from build123d import *

# Parameters (mm, degrees)
SKETCH1_R           = 5
SKETCH1_R_2         = 2
SKETCH1_R_3         = 4
SKETCH1_R_4         = 11
BOSS_EXTRUDE1_DEPTH = 6


with BuildPart() as part:
    # Sketch1 → Boss-Extrude1 (new body)
    with BuildSketch(Plane.XY):
        with BuildLine():
            Line((-91.133667709, 81.856650449), (-59.395664216, 82.872754588))
            ThreePointArc((-59.395664216, 82.872754588), (-54.441095215, 84.371809376), (-50.89983999, 88.147313406))
            Line((-50.89983999, 88.147313406), (49.994476852, 276.580618392))
            Line((49.994476852, 276.580618392), (30.200235156, 308.463550017))
            ThreePointArc((30.200235156, 308.463550017), (26.424731127, 312.004805242), (21.384421113, 313.183870213))
            Line((21.384421113, 313.183870213), (-16.12412847, 311.983019868))
            Line((-16.12412847, 311.983019868), (-117.018445312, 123.549714881))
            ThreePointArc((-117.018445312, 123.549714881), (-118.197510284, 118.509404868), (-116.698455495, 113.554835867))
            Line((-116.698455495, 113.554835867), (-99.949481752, 86.576970646))
            ThreePointArc((-99.949481752, 86.576970646), (-96.173977723, 83.035715421), (-91.133667709, 81.856650449))
        make_face()
        with Locations((1.104829999, 270.012836125)):
            Circle(SKETCH1_R, mode=Mode.SUBTRACT)
        with Locations((-33.33250289, 254.422130449)):
            Circle(SKETCH1_R_2, mode=Mode.SUBTRACT)
        with Locations((11.628148729, 230.348497445)):
            Circle(SKETCH1_R_2, mode=Mode.SUBTRACT)
        with Locations((-28.022540924, 156.295659484)):
            Circle(SKETCH1_R_2, mode=Mode.SUBTRACT)
        with Locations((-43.879665152, 180.702169371)):
            Circle(SKETCH1_R_3, mode=Mode.SUBTRACT)
        with Locations((-72.983192543, 180.369292488)):
            Circle(SKETCH1_R_2, mode=Mode.SUBTRACT)
        with Locations((-76.464627777, 119.845498823)):
            Circle(SKETCH1_R_4, mode=Mode.SUBTRACT)
    extrude(amount=BOSS_EXTRUDE1_DEPTH)


solid = part.part
The model under review builds one solid part; all positions refer to its coordinate system, in mm. Coordinates: 2 decimals unless noted, no trailing zeros. Write each loop counter-clockwise with the first axis right and the second up, starting at its lowest first coordinate (ties: lowest second). Pieces come first, ordered by that corner, then holes. Notation, with made-up numbers: M 12.5,-12.5 L 54.5,-12.5 A19 cw 54.5,14.5 Z; hole C 2.25,47.25 d7. An arc over 180 degrees is marked long. Put each result on its own line as item: value.
1) Draft analysis for pull direction Z (two halves, no side actions). For faces 1 (the flat face through (-35, 199, 0)), 2 (the cylindrical face through (-65.973, 123.15, 2.958)), 3 (the flat face through (-35, 199, 6)), state which applies: released by +Z, released by -Z, zero draft, split by the parting line, or undercut.
Computed:
face 1: released by -Z
face 2: zero draft
face 3: released by +Z
2) Wall thickness on probe 1 along X at (y, z) = (231.5, 0.5); probe 2 along X at (y, z) = (116.5, 2.15); probe 3 along Y at (x, z) = (11, 1.4): over which ranges is each line inside the solid? List them lowest first. Write a range as [from, to].
Computed:
probe 1: x = [-59.22, 9.99], [13.26, 25.86]
probe 2: x = [-117.93, -86.94], [-65.99, -35.72]
probe 3: y = [203.75, 228.45], [232.25, 312.85]
3) Add section A-A on x = -43.5. Give the boundary of the cut face in (y, z) (3 decimals).
Computed:
outline: M 101.967,0 L 176.72,0 L 176.72,6 L 101.967,6 Z; M 184.684,0 L 260.855,0 L 260.855,6 L 184.684,6 Z
4) Clearance check with flat-ended pins moving along their axes: pin 1 Ø3 at (x, z) = (-54, 5) entering from -Y; pin 2 Ø1 at (x, z) = (6, 1.5) entering from -Y; pin 3 Ø1 at (y, z) = (106, 4) entering from -X. State where each tip first meets the part, or that it passes through.
Computed:
pin 1: stops at y = 83.8
pin 2: stops at y = 193.48
pin 3: stops at x = -112.32
5) Add section B-B on z = 2.75. Give the boundary of the cut face in (x, y).
Computed:
outline: M -117.02,123.55 A10 ccw -116.7,113.55 L -99.95,86.58 A10 ccw -91.13,81.86 L -59.4,82.87 A10 ccw -50.9,88.15 L 49.99,276.58 L 30.2,308.46 A10 ccw 21.38,313.18 L -16.12,311.98 Z; hole C -76.46,119.85 d22; hole C -72.98,180.37 d4; hole C -43.88,180.7 d8; hole C -33.33,254.42 d4; hole C -28.02,156.3 d4; hole C 1.1,270.01 d10; hole C 11.63,230.35 d4
6) Add section D-D on y = 196.5. Give the boundary of the cut face in (x, z).
Computed:
outline: M -77.96,0 L 7.12,0 L 7.12,6 L -77.96,6 Z
7) Add section C-C on x = -77.5. Give the boundary of the cut face in (y, z), then the cut area to 3 significant figures.
Computed:
outline: M 82.29,0 L 108.89,0 L 108.89,6 L 82.29,6 Z; M 130.8,0 L 197.36,0 L 197.36,6 L 130.8,6 Z
area: 559 mm2
